The listing builds one solid part. Answer for the finished solid, in the listing's coordinates (mm). Face numbers are marked on the shaded views. A direction names the side the tool comes from. Give positions to 0.01 mm unless a question says otherwise; leave off trailing zeros. Order: outer loops, then holes, each group sorted by start corner. A loop starts at its lowest first (then second) coordinate and runs counter-clockwise, first axis right, second up. Notation, with made-up numbers: (-5.5, 39) - (48.5, 39) arc R23 cw to (48.5, 55) - close; hole circle Ø7 at (54.25, 67). An arc over 180 degrees is marked (long way). Answer as CSV lines item,"result". Start each with the question number.
1. Determine the mould class of the marked faces 1, 2 and 3 for opening direction Y: +Y half, -Y half, draft (parallel to the pull), parting line (faces both ways), or undercut.
2. Consider line 1 along Y through (x, z) = (-3, 5.75); line 2 along Y through (x, z) = (-3.25, 1.5); line 3 along X through (y, z) = (-0.75, 6.5). Determine where each line is inside the solid, lowest interval first. Write a range as [from, to].
3. Which of the six approach directions +Z, -Z, +X, -X, +Y, -Y give full straight-line access (tool end or side, diameter ignored) to the marked faces 4, 5 and 6?
4. Section D-D on y = -0.5 is taken. Give the vertices of the cut face in (x, z), and give its area (3 significant figures).
5. Flat-ended cylindrical pins translate along their axes: pin 1 (0.6 mm diameter, centred on y = 0, z = 6.5, fed in from +X); pin 2 (0.6 mm diameter, centred on y = -0.5, z = 7.5, fed in from -X); pin 3 (1.5 mm diameter, centred on y = 1, z = 2.5, fed in from +X). Find the tip coordinate at first contact, or state that the pin passes through.
6. Section C-C on x = 0 is taken. Give the vertices of the cut face in (y, z), and give its area (3 significant figures).
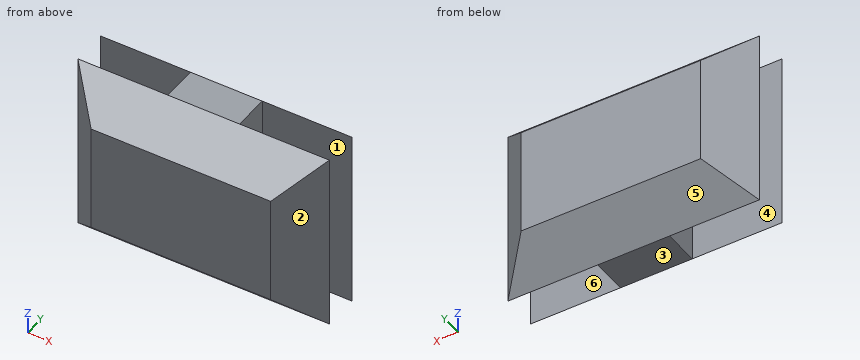
from build123d import *

# Parameters (mm, degrees)
F0_W     = 4
F0_H     = 2
F1_DEPTH = 10
F2_SIZE  = 1.99999
F3_SIZE  = 1.99999


# Not quite as in the source:
# - a fillet or chamfer is up to 0.001 mm smaller than in the source, because OpenCascade refuses the exact size


with BuildPart() as f1:
    # F0 (on Top) → F1 (new body)
    with BuildSketch(Plane.XY):
        Polygon((-7, 3), (-7, 1), (-2, 1), (2, 1), (7, 1), (7, 3), align=None)
        Rectangle(F0_W, F0_H)
        Polygon((-2, -1), (-7, -1), (-7, -3), (7, -3), (7, -1), (2, -1), align=None)
    extrude(amount=F1_DEPTH)

    # F2 (size 2 in the source; OpenCascade refuses exactly that, so slightly less here)
    f2_edges = [f1.edges().sort_by_distance(p)[0] for p in [
        (-7, 3, 5),
        (7, 3, 5),
        (7, -3, 5),
        (-7, -3, 5),
    ]]
    chamfer(f2_edges, length=F2_SIZE)

    # F3 (size 2 in the source; OpenCascade refuses exactly that, so slightly less here)
    f3_edges = [f1.edges().sort_by_distance(p)[0] for p in [
        (0, 3, 10),
        (0, -3, 10),
        (0, -3, 0),
        (0, 3, 0),
    ]]
    chamfer(f3_edges, length=F3_SIZE)


solid = f1.part
Checks:
1,face 1,"undercut"
1,face 2,"-Y half"
1,face 3,"draft"
2,line 1,"y = [-3, -1], [1, 3]"
2,line 2,"y = [-2.5, -1], [1, 2.5]"
2,line 3,"x = [-2, 2]"
3,face 4,"+Z, -Z, -X"
3,face 5,"-Z, +X, -X, +Y"
3,face 6,"+Z, -Z, +X"
4,outline,"(-2, 0) - (2, 0) - (2, 10) - (-2, 10) - close"
4,area,"40.0 mm²"
5,pin 1,"stops at x = 2"
5,pin 2,"stops at x = -2"
5,pin 3,"stops at x = 7"
6,outline,"(-3, 2) - (-1, 0) - (1, 0) - (3, 2) - (3, 8) - (1, 10) - (-1, 10) - (-3, 8) - close"
6,area,"52.0 mm²"
